Verification items for the finished model (mm, model axes). A direction names the side the tool comes from. Round coordinates to 2 decimals unless told otherwise and drop trailing zeros. Write each loop counter-clockwise with the first axis right and the second up, starting at its lowest first coordinate (ties: lowest second). Pieces come first, ordered by that corner, then holes. Notation, with made-up numbers: (6, 49.5) -> (18, 49.5) arc R21 cw to (18, 63.5) -> close; hole circle Ø11 at (-29, 65.5). An arc over 180 degrees is marked (long way). Use CSV: the item, a comma, the result in double quotes.
Autodesk Inventor part; units mm, degrees
ref_plane "YZ Plane" through (0, 0, 0) normal (1, 0, 0) x (0, 1, 0)
ref_plane "XZ Plane" through (0, 0, 0) normal (0, 1, 0) x (-1, 0, 0)
ref_plane "XY Plane" through (0, 0, 0) normal (0, 0, 1) x (1, 0, 0)
sketch "Sketch1" plane through (0, 0, 0) normal (1, 0, 0) x (0, 1, 0)
  line L0 (1.5, -5) -> (1.5, 5)
  line L1 (1.5, 5) -> (-7.7318, 5)
  line L2 (-9.4639, 2) -> (-1.5, 2)
  line L3 (-1.5, 2) -> (-1.5, -5)
  line L4 (-1.5, -5) -> (1.5, -5)
  line L5 (-7.7318, 5) -> (-27.7318, 39.641)
  line L6 (-27.7318, 39.641) -> (-30.3299, 38.141)
  line L7 (-30.3299, 38.141) -> (-9.4639, 2)
  point P0 (0, 0)
  point P1 (0, -5)
  point P2 (1.5, 0)
  dimension "d0" = 3
  dimension "d1" = 10
  dimension "d2" = 150
  dimension "d3" = 3
  dimension "d4" = 3
  dimension "d5" = 40
  dimension "d6" = 7.995
extrude "Extrusion1" add sketch "Sketch1" along normal mid plane 40
fillet "Fillet1" radius 3.5 2 edges at (0, 1.5, 5) (0, -9.4639, 2)
fillet "Fillet1" radius 0.5 2 edges at (0, -1.5, 2) (0, -7.7318, 5)
sketch "Sketch2" plane through (-20, -1.5, -5) normal (0, -1, 0) x (1, 0, 0)
  line L0 (30, 3.5) -> (10, 3.5) construction
  line L1 (0, 0) -> (40, 0) construction
  point P0 (20, 5)
  point P1 (20, 3.5)
  dimension "d11" = 20
  dimension "d12" = 3.5
hole "Hole1" at (10, -1.5, -1.5) at (-10, -1.5, -1.5) direction (0, 1, 0) diameter 3.3 end through all
sketch "Sketch3" plane through (-20, -27.7318, 39.641) normal (0, 0.8660254, 0.5) x (1, 0, 0)
  line L0 (0, 39.7113) -> (40, 39.7113)
  line L1 (0, 0) -> (0, 39.7113)
  line L2 (0, 0) -> (40, 0)
  line L3 (40, 39.7113) -> (40, 0)
  line L4 (0, 0) -> (40, 0)
  line L5 (10, 0) -> (0, 36.7113)
  line L6 (0, 39.7113) -> (0, 0)
  line L7 (40, 36.7113) -> (30, 0)
  circle A0 centre (10, 34.7113) radius 3.5
  circle A1 centre (30, 34.7113) radius 3.5
  line L8 (10, 34.7113) -> (30, 34.7113) construction
  point P0 (20, 48.196)
  point P1 (20, 34.7113)
  point P2 (20, 0)
  dimension "d20" = 7
  dimension "d21" = 20
  dimension "d22" = 3
  dimension "d23" = 20
  dimension "d24" = 5
extrude "Extrusion2" cut sketch "Sketch3" against normal through all contours L5 L2 L1 | L3 L2 L7 | A0 | A1
equation "\"d3\" = d0"
equation "\"d4\" = d0"
properties part number "P-POD_DoorStop" material "Aluminum 6061"
Q1. Go/stop test with flat-tipped pins: P1, Ø4, axis at x = 10, z = -1.5, coming from the +Y side; P2, Ø12, axis at x = 7.5, z = 15, coming from the -Y side; P3, Ø8, axis at x = 11, z = 3, coming from the -Y side; P4, Ø2.5, axis at x = 5, y = -4.5, coming from the -Z side. Record where each tip stops, or that it passes through.
Filled in:
P1,"y = 1.5"
P2,"y = -20.43"
P3,"y = -12.05"
P4,"z = 2"
Q2. Section check A-A (x = 1.5). Record the cut outline in (y, z).
Filled in:
outline,"(-30.33, 38.14) -> (-10.47, 3.75) arc R3.5 ccw to (-7.44, 2) -> (-2, 2) arc R0.5 cw to (-1.5, 1.5) -> (-1.5, -5) -> (1.5, -5) -> (1.5, 1.5) arc R3.5 ccw to (-2, 5) -> (-7.44, 5) arc R0.5 cw to (-7.88, 5.25) -> (-27.73, 39.64) -> close"
Q3. Material ranges on L1, parallel to X at y = -0.8, z = -1.5; L2, parallel to Z at x = -17, y = -7; L3, parallel to Z at x = -10, y = 0, recorded low to high.
Filled in:
L1,"-20 to -11.65, -8.35 to 8.35, 11.65 to 20"
L2,"2 to 5"
L3,"-5 to -3.15, 0.15 to 4.37"
Q4. Section check B-B (y = -6). Record the cut outline in (x, z).
Filled in:
outline,"(-20, 2) -> (20, 2) -> (20, 5) -> (-20, 5) -> close"
Q5. Mould release check, pull along Z, two halves, no side actions. Record for faces 1 (the flat face through (0, -5, 5)), 2 (the cylindrical face through (13.233, -12.327, 10.002)), 3 (the flat face through (0, 0, -5)): released by +Z, released by -Z, zero draft, split by the parting line, or undercut.
Filled in:
face 1,"released by +Z"
face 2,"undercut"
face 3,"released by -Z"
Q6. Access from +Z, -Z, +X, -X, +Y, -Y to the whole of each face (thin tool, end or side, straight path). Record for faces 4 (the flat face through (0, -1.5, -2)), 5 (the flat face through (-20, -3.8, 2.4)).
Filled in:
face 4,"-Z, +X, -X, -Y"
face 5,"+Z, -Z, -X, +Y, -Y"
Q7. Section check C-C (y = -21). Record the cut outline in (x, z), plus the area to 3 significant figures.
Filled in:
outline,"(-15.08, 21.98) -> (15.08, 21.98) -> (13.67, 27.98) -> (-13.67, 27.98) -> close"
area,"173 mm²"
